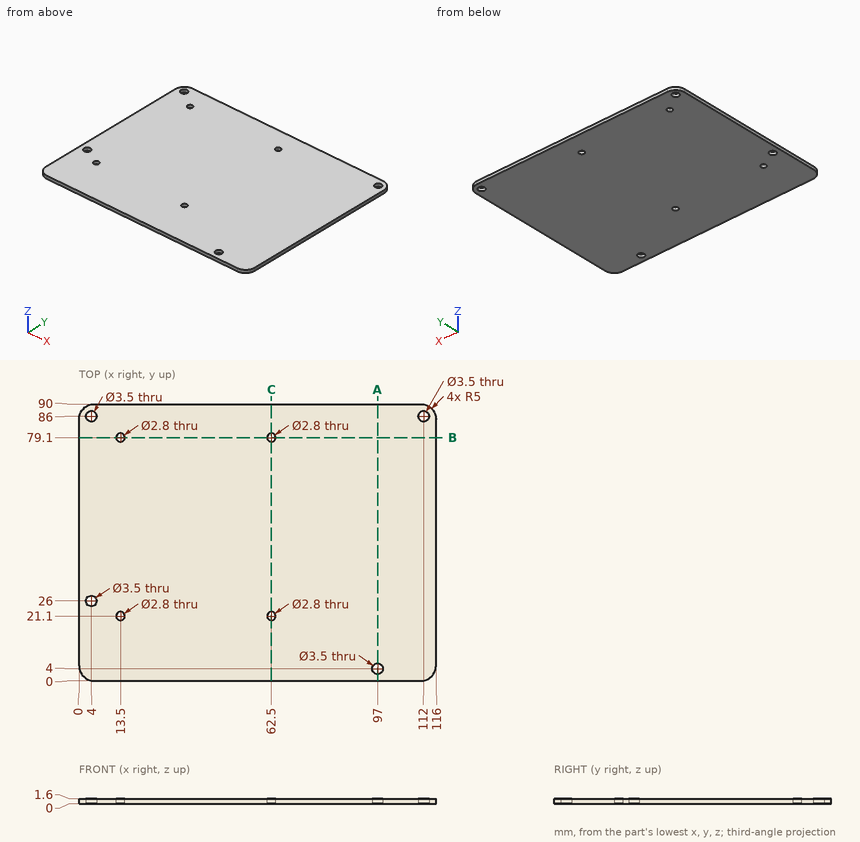
Verification items for this drawing (mm, ordinates from the low corner). Coordinates: 2 decimals unless noted, no trailing zeros. Loops run counter-clockwise (first coordinate to the right, second up) from the corner with the lowest first, then second, coordinate; pieces in that order, holes last. Notation, with made-up numbers: (32.25, 11) -> (64.25, 11) arc R6 ccw to (64.25, 18) -> close; hole circle Ø10 at (3.25, -10.5). An arc over 180 degrees is marked (long way). Put each result on its own line as item: value.
1. Section check A-A, the plane x = 97. Record the boundary of the cut face in (y, z).
Result set:
outline: (0, 0) -> (2.25, 0) -> (2.25, 1.6) -> (0, 1.6) -> close; (5.75, 0) -> (90, 0) -> (90, 1.6) -> (5.75, 1.6) -> close
2. Section check C-C, the plane x = 62.5. Record the boundary of the cut face in (y, z).
Result set:
outline: (0, 0) -> (19.7, 0) -> (19.7, 1.6) -> (0, 1.6) -> close; (22.5, 0) -> (77.7, 0) -> (77.7, 1.6) -> (22.5, 1.6) -> close; (80.5, 0) -> (90, 0) -> (90, 1.6) -> (80.5, 1.6) -> close
3. Gauge pin test, flat end, axial feed: P1, Ø3, axis at x = 13.5, y = 21.1, coming from the -Z side. Record the tip position at first contact, or that the pin passes through.
Result set:
P1: stops at z = 0
4. Thickness scan on line 1 (Y direction, x = 13.5, z = 0.65); line 2 (X direction, y = 79.1, z = 0.8); line 3 (Y direction, x = 4, z = 0.5). Record the ranges inside material, lowest first.
Result set:
line 1: y = 0 to 19.7, 22.5 to 77.7, 80.5 to 90
line 2: x = 0 to 12.1, 14.9 to 61.1, 63.9 to 116
line 3: y = 0.1 to 24.25, 27.75 to 84.25, 87.75 to 89.9
5. Section check B-B, the plane y = 79.1. Record the boundary of the cut face in (x, z).
Result set:
outline: (0, 0) -> (12.1, 0) -> (12.1, 1.6) -> (0, 1.6) -> close; (14.9, 0) -> (61.1, 0) -> (61.1, 1.6) -> (14.9, 1.6) -> close; (63.9, 0) -> (116, 0) -> (116, 1.6) -> (63.9, 1.6) -> close
